from build123d import *

# Parameters (mm, degrees)
SKETCH1_W            = 31.5
SKETCH1_H            = 52.5
BASE_FLANGE1_DEPTH   = 3
EDGE_FLANGE1_DEPTH   = 31.5
EDGE_FLANGE2_DEPTH   = 52.5
CUT_EXTRUDE1_DEPTH   = 10
M4_CLEARANCE_HOLE1_D = 4.3
M4_CLEARANCE_HOLE2_D = 4.3


# Sheet-metal steps are written as plain solids
with BuildPart() as part:
    # Sketch1 → Base-Flange1 (new body)
    with BuildSketch(Plane(origin=(0, 0, 0), x_dir=(1, 0, 0), z_dir=(0, 1, 0))):
        with Locations((-15.75, 26.25)):
            Rectangle(SKETCH1_W, SKETCH1_H)
    extrude(amount=-BASE_FLANGE1_DEPTH)

    # Edge-Flange1 section (across the edge) → Edge-Flange1 (add)
    with BuildSketch(Plane(origin=(0, -3, 2.5), x_dir=(0, 0, -1), z_dir=(-1, 0, 0))):
        with BuildLine():
            Line((-3, 2.5), (-3, 19))
            Line((-3, 19), (0, 19))
            Line((0, 19), (0, 2.5))
            ThreePointArc((0, 2.5), (0.732233047, 0.732233047), (2.5, 0))
            Line((2.5, 0), (2.5, -3))
            ThreePointArc((2.5, -3), (-1.389087297, -1.389087297), (-3, 2.5))
        make_face()
    extrude(amount=EDGE_FLANGE1_DEPTH)

    # Edge-Flange2 section (across the edge) → Edge-Flange2 (add)
    with BuildSketch(Plane(origin=(-34, -3, 0), x_dir=(1, 0, 0), z_dir=(0, 0, -1))):
        with BuildLine():
            Line((-3, 2.5), (-3, 19))
            Line((-3, 19), (0, 19))
            Line((0, 19), (0, 2.5))
            ThreePointArc((0, 2.5), (0.732233047, 0.732233047), (2.5, 0))
            Line((2.5, 0), (2.5, -3))
            ThreePointArc((2.5, -3), (-1.389087297, -1.389087297), (-3, 2.5))
        make_face()
    extrude(amount=EDGE_FLANGE2_DEPTH)

    # Sketch12 → Cut-Extrude1 (cut)
    with BuildSketch(Plane(origin=(0, 0, 0), x_dir=(1, 0, 0), z_dir=(0, 1, 0))):
        Polygon((-31.5, 52.5), (0, 0), (0, 52.5), align=None)
    extrude(amount=-CUT_EXTRUDE1_DEPTH, mode=Mode.SUBTRACT)

    # M4 Clearance Hole1 (through all)
    with Locations(Plane(origin=(0, 0, 2.5), x_dir=(-1, 0, 0), z_dir=(0, 0, -1))):
        with Locations((7, -13.5), (25, -13.5)):
            Hole(M4_CLEARANCE_HOLE1_D / 2)

    # M4 Clearance Hole2 (through all)
    with Locations(Plane(origin=(-34, 0, 0), x_dir=(0, 0, -1), z_dir=(1, 0, 0))):
        with Locations((44.5, -13.5), (8.5, -13.5)):
            Hole(M4_CLEARANCE_HOLE2_D / 2)


solid = part.part
Could you check a few things on this model? Use its own coordinates, in mm. A direction names the side the tool comes from. Round coordinates to 2 decimals unless told otherwise and drop trailing zeros. Order: outer loops, then holes, each group sorted by start corner. A loop starts at its lowest first (then second) coordinate and runs counter-clockwise, first axis right, second up.
Q1. Imagine slicing it at B-B, the plane y = -17.75. List the corners of the cut face in (x, z) for me, then the cut area to 3 significant figures.
Geometry says:
outline: (-37, -52.5) - (-34, -52.5) - (-34, 0) - (-37, 0) - close; (-31.5, 2.5) - (0, 2.5) - (0, 5.5) - (-31.5, 5.5) - close
area: 252 mm2
Q2. Imagine slicing it at C-C, the plane x = -8. List the corners of the cut face in (y, z) for me, then the cut area to 3 significant figures.
Geometry says:
outline: (-22, 2.5) - (-15.4, 2.5) - (-15.4, 5.5) - (-22, 5.5) - close; (-11.6, 2.5) - (-5.5, 2.5) arc R2.5 cw to (-3, 0) - (-3, -13.33) - (0, -13.33) - (0, 0) arc R5.5 ccw to (-5.5, 5.5) - (-11.6, 5.5) - close
area: 96.9 mm2
Q3. Imagine slicing it at A-A, the plane z = -8.5. List the corners of the cut face in (x, y) for me, then the cut area to 3 significant figures.
Geometry says:
outline: (-37, -22) - (-34, -22) - (-34, -15.65) - (-37, -15.65) - close; (-37, -11.35) - (-34, -11.35) - (-34, -5.5) arc R2.5 cw to (-31.5, -3) - (-5.1, -3) - (-5.1, 0) - (-31.5, 0) arc R5.5 ccw to (-37, -5.5) - close
area: 135 mm2
Q4. Imagine slicing it at D-D, the plane x = -30. List the corners of the cut face in (y, z) for me, then the cut area to 3 significant figures.
Geometry says:
outline: (-22, 2.5) - (-5.5, 2.5) arc R2.5 cw to (-3, 0) - (-3, -50) - (0, -50) - (0, 0) arc R5.5 ccw to (-5.5, 5.5) - (-22, 5.5) - close
area: 218 mm2
Q5. Please list where these lines run through material, in increasing order: probe 1 along X at (y, z) = (-11.25, -14.5); probe 2 along Z at (x, y) = (-16.5, -16.5); probe 3 along Y at (x, z) = (-17, -11.5).
Geometry says:
probe 1: x = -37 to -34
probe 2: z = 2.5 to 5.5
probe 3: y = -3 to 0
Q6. Which directions (+Z, -Z, +X, -X, +Y, -Y) give clear straight access to the entire face, cutting with the end or side of a thin tool? Please do faces 4 (the face through (-23, -3, -15)), 5 (the face through (-16, -14, 2.5)), 6 (the face through (-33.287, -3.752, -25.882)), 7 (the face through (-16, -14, 5.5)), 8 (the face through (-31.5, -11, 3)).
Geometry says:
face 4: -Z, +X, -Y
face 5: -Z, +X, -X, -Y
face 6: +Z, -Z, +X, -Y
face 7: +Z, +X, -X, +Y, -Y
face 8: +Z, -X, +Y, -Y
Q7. I'm going to push flat-ended pins straight in: P1, Ø5, axis at x = -8.5, y = -11.5, coming from the -Z side; P2, Ø10, axis at x = -11.5, z = -36.5, coming from the -Y side; P3, Ø1.5, axis at y = -12, z = -1.5, coming from the +X side; P4, Ø16, axis at x = -21, z = -18.5, coming from the -Y side. Where does each tip first touch, or does it pass through?
Geometry says:
P1: stops at z = 2.5
P2: passes through
P3: stops at x = -34
P4: stops at y = -3
Q8. Thinking about a two-plate mould opening in Y: for faces 1 (the face through (-35.35, -1.57, -25.88)), 2 (the face through (-35.521, -14.323, -42.514)), 3 (the face through (-34, -14, -26)), which applies, released by +Y, released by -Y, zero draft, split by the parting line, or undercut?
Geometry says:
face 1: released by +Y
face 2: undercut
face 3: zero draft
